```python
from build123d import *

# Parameters (mm, degrees)
SKETCH_1_R      = 1.5
EXTRUDE_1_DEPTH = 1.5
FILLET_1_R      = 5


with BuildPart() as part:
    # 草图1 → 凸台-拉伸1 (new, symmetric)
    with BuildSketch(Plane.XY):
        Polygon((0, 40), (0, -40), (21, -40), (60, -13), (60, 13), (21, 40), align=None)
        with Locations((10, 0)):
            Circle(SKETCH_1_R, mode=Mode.SUBTRACT)
        with Locations((10, 15)):
            Circle(SKETCH_1_R, mode=Mode.SUBTRACT)
        with Locations((10, 30)):
            Circle(SKETCH_1_R, mode=Mode.SUBTRACT)
        with Locations(Location((10, -15, 0), (0, 0, 180))):
            Circle(SKETCH_1_R, mode=Mode.SUBTRACT)
        with Locations(Location((10, -30, 0), (0, 0, 180))):
            Circle(SKETCH_1_R, mode=Mode.SUBTRACT)
        with Locations((30, 0)):
            Circle(SKETCH_1_R, mode=Mode.SUBTRACT)
        with Locations((40, 0)):
            Circle(SKETCH_1_R, mode=Mode.SUBTRACT)
        with Locations((50, 0)):
            Circle(SKETCH_1_R, mode=Mode.SUBTRACT)
    extrude(amount=EXTRUDE_1_DEPTH, both=True)

    # 圆角1
    fillet_1_edges = [part.edges().sort_by_distance(p)[0] for p in [
        (60, 13, 0),
        (60, -13, 0),
        (21, -40, 0),
        (21, 40, 0),
    ]]
    fillet(fillet_1_edges, radius=FILLET_1_R)


solid = part.part
```
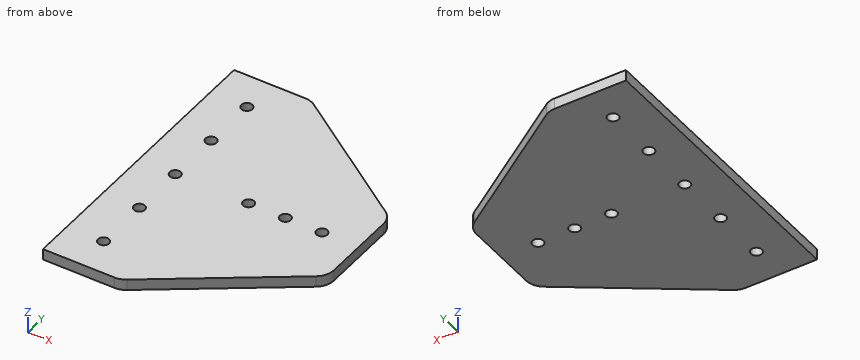
Check sheet for the modelled part. Datum: model origin and axes. Units: mm. Coordinates: 2 decimals unless noted, no trailing zeros. Order: outer loops, then holes, each group sorted by start corner. A loop starts at its lowest first (then second) coordinate and runs counter-clockwise, first axis right, second up. Notation, with made-up numbers: M 77,16.25 L 114,16.25 A11 cw 114,32.25 Z; hole C -39.75,32.5 d4. An arc over 180 degrees is marked long. Write each question's results on one line, items separated by ' | '. Start each with the question number.
1. Cross-section at A-A on x = 10. Record the cut outline in (y, z).
2. Cross-section at D-D on x = 50. Record the cut outline in (y, z).
3. Cross-section at C-C on z = -1.05. State how many separate pieces and enclosed holes the cut face has, and give its area (3 significant figures).
4. Material ranges on probe 1 along Y at (x, z) = (10, -0.35); probe 2 along Y at (x, z) = (50, -0.75); probe 3 along Y at (x, z) = (40, 0.55), recorded low to high.
5. Go/stop test with flat-tipped pins: P1, Ø2.5, axis at x = 30, y = 0, coming from the -Z side; P2, Ø1, axis at x = 41.5, z = -1, coming from the +Y side; P3, Ø1, axis at y = 25, z = -1, coming from the +X side. Record where each tip stops, or that it passes through.
6. Cross-section at B-B on y = -30. Record the cut outline in (x, z).
Checks:
1) outline: M -40,-1.5 L -31.5,-1.5 L -31.5,1.5 L -40,1.5 Z; M -28.5,-1.5 L -16.5,-1.5 L -16.5,1.5 L -28.5,1.5 Z; M -13.5,-1.5 L -1.5,-1.5 L -1.5,1.5 L -13.5,1.5 Z; M 1.5,-1.5 L 13.5,-1.5 L 13.5,1.5 L 1.5,1.5 Z; M 16.5,-1.5 L 28.5,-1.5 L 28.5,1.5 L 16.5,1.5 Z; M 31.5,-1.5 L 40,-1.5 L 40,1.5 L 31.5,1.5 Z
2) outline: M -19.92,-1.5 L -1.5,-1.5 L -1.5,1.5 L -19.92,1.5 Z; M 1.5,-1.5 L 19.92,-1.5 L 19.92,1.5 L 1.5,1.5 Z
3) separate pieces: 1 | enclosed holes: 8 | area: 3,690 mm²
4) probe 1: y = -40 to -31.5, -28.5 to -16.5, -13.5 to -1.5, 1.5 to 13.5, 16.5 to 28.5, 31.5 to 40 | probe 2: y = -19.92 to -1.5, 1.5 to 19.92 | probe 3: y = -26.85 to -1.5, 1.5 to 26.85
5) P1: passes through | P2: stops at y = 26.15 | P3: stops at x = 43.39
6) outline: M 0,-1.5 L 8.5,-1.5 L 8.5,1.5 L 0,1.5 Z; M 11.5,-1.5 L 35.44,-1.5 L 35.44,1.5 L 11.5,1.5 Z
